Print and shaded views of the part. All mm, measured from the part's lowest x, y and z. A direction names the side the tool comes from. Coordinates: 2 decimals unless noted, no trailing zeros. Loops run counter-clockwise (first coordinate to the right, second up) from the corner with the lowest first, then second, coordinate; pieces in that order, holes last. Notation, with made-up numbers: M -36,1.5 L 23,1.5 A26 ccw 23,34.5 Z; hole C 21.5,-4 d2. An arc over 180 degrees is marked long. Use a Markdown table: item, result. Add a question column.
1) Pin check, flat tips, straight feed: pin 1 Ø1.8 at (x, z) = (9, 3.5) entering from +Y; pin 2 Ø2 at (y, z) = (54, 3) entering from +X; pin 3 Ø1.8 at (y, z) = (2.5, 4) entering from -X. Stop position of each tip, or through.
2) Band-saw the part on D-D (x = 4.5). List the corners of the cut face in (y, z), plus the area to 3 significant figures.
3) Tool access for the marked faces 1, 2 and 3: list every direction of +Z, -Z, +X, -X, +Y, -Y with a clear straight run to the whole face (end or side of a thin tool).
4) Band-saw the part on A-A (x = 8). List the corners of the cut face in (y, z).
5) Wall check: probe 1 along Y at (x, z) = (8.5, 4); probe 2 along Z at (x, y) = (1.05, 54); probe 3 along Y at (x, z) = (7.5, 1.6). Give the ranges that are in metal, low to high. Write a range as from..to.
6) Band-saw the part on C-C (y = 43). List the corners of the cut face in (x, z), plus the area to 3 significant figures.
7) Band-saw the part on B-B (z = 0.8). List the corners of the cut face in (x, y).
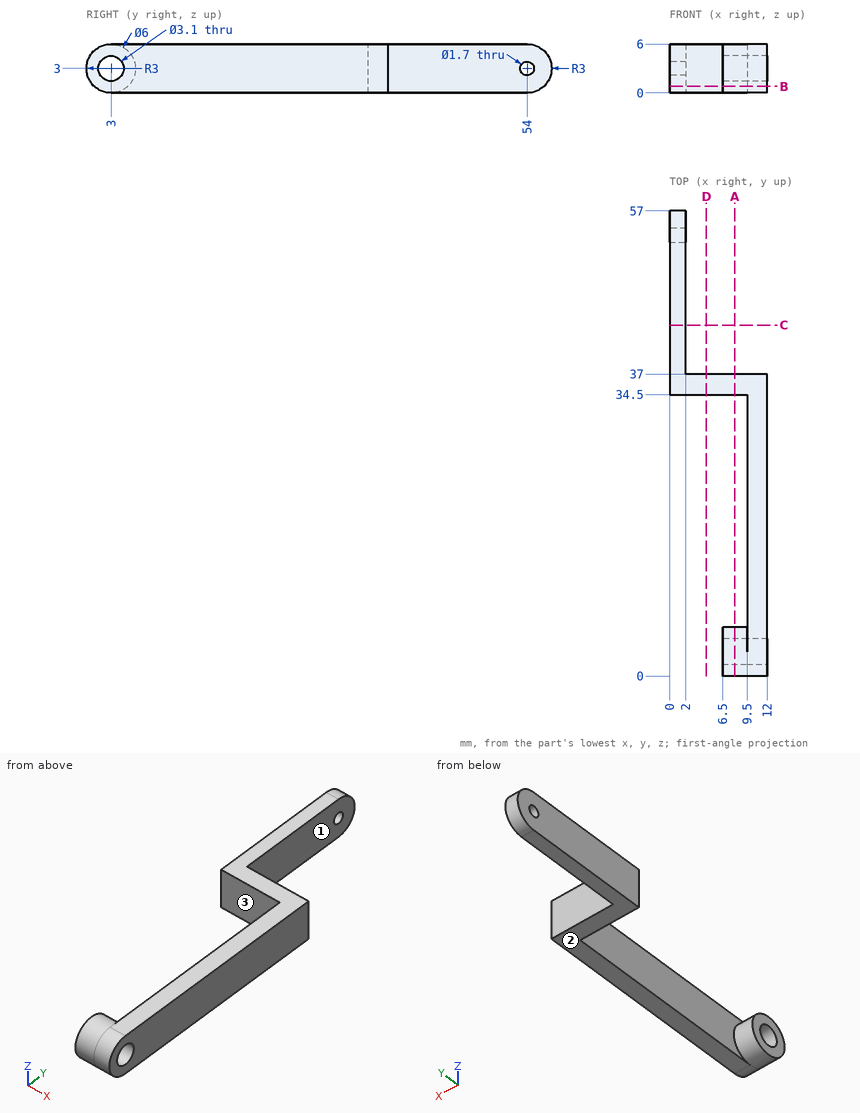
Entries:
| question | item | result |
|---|---|---|
| 1 | pin 1 | y = 37 |
| 1 | pin 2 | x = 2 |
| 1 | pin 3 | x = 6.5 |
| 2 | outline | M 34.5,0 L 37,0 L 37,6 L 34.5,6 Z |
| 2 | area | 15.0 mm2 |
| 3 | face 1 | +Z, -Z, +X, +Y |
| 3 | face 2 | -Z, +X, -X, +Y, -Y |
| 3 | face 3 | +Z, -Z, -X |
| 4 | outline | C 3,3 d6; M 34.5,0 L 37,0 L 37,6 L 34.5,6 Z; hole C 3,3 d3.1 |
| 5 | probe 1 | 0.17..1.82, 4.18..5.83, 34.5..37 |
| 5 | probe 2 | 0..2.15, 3.85..6 |
| 5 | probe 3 | 0.35..2.33, 3.67..5.65, 34.5..37 |
| 6 | outline | M 0,0 L 2,0 L 2,6 L 0,6 Z |
| 6 | area | 12.0 mm2 |
| 7 | outline | M 0,34.5 L 9.5,34.5 L 9.5,5.04 L 6.5,5.04 L 6.5,0.96 L 12,0.96 L 12,37 L 2,37 L 2,56.04 L 0,56.04 Z |
